```python
from build123d import *

# Parameters (mm, degrees)
CROQUIS1_R                                           = 1.5
CROQUIS1_R_2                                         = 1.75
CROQUIS1_W                                           = 8.011123414
CROQUIS1_H                                           = 3.391601998
CROQUIS1_R_3                                         = 1.642596358
SALIENTE_EXTRUIR1_DEPTH                              = 5
REFRENTADO_PARA_TORNILLO_TAP_N_CON_CABEZ_D           = 3.2
REFRENTADO_PARA_TORNILLO_TAP_N_CON_CABEZ_CSINK_D     = 4.72
REFRENTADO_PARA_TORNILLO_TAP_N_CON_CABEZ_CSINK_ANGLE = 90
REFRENTADO_PARA_TORNILLO_TAP_N_CON_C_2_D             = 3.2
REFRENTADO_PARA_TORNILLO_TAP_N_CON_C_2_CSINK_D       = 6.72
REFRENTADO_PARA_TORNILLO_TAP_N_CON_C_2_CSINK_ANGLE   = 90
CROQUIS7_W                                           = 8
CROQUIS7_H                                           = 13.5
CORTAR_EXTRUIR1_DEPTH                                = 3
CROQUIS8_W                                           = 8
CROQUIS8_H                                           = 2.993534549
CORTAR_EXTRUIR2_DEPTH                                = 10


with BuildPart() as part:
    # Croquis1 → Saliente-Extruir1 (new body)
    with BuildSketch(Plane(origin=(0, 0, 0), x_dir=(1, 0, 0), z_dir=(0, 1, 0))):
        Polygon((-26, 8.5), (-50, 8.5), (-50, -37.5), (50, -37.5), (50, 8.5), (26, 8.5), (26, 37.5), (-26, 37.5), align=None)
        with Locations(Location((-47.484488335, -31.135629499, 0), (0, 0, 270))):
            Circle(CROQUIS1_R, mode=Mode.SUBTRACT)
        with Locations(Location((-47.484488335, -18.135629499, 0), (0, 0, 270))):
            Circle(CROQUIS1_R, mode=Mode.SUBTRACT)
        with Locations(Location((0, -9.329285485, 0), (0, 0, 270))):
            Circle(CROQUIS1_R_2, mode=Mode.SUBTRACT)
        with Locations(Location((47.484488335, -31.135629499, 0), (0, 0, 270))):
            Circle(CROQUIS1_R, mode=Mode.SUBTRACT)
        with Locations(Location((47.484488335, -18.135629499, 0), (0, 0, 270))):
            Circle(CROQUIS1_R, mode=Mode.SUBTRACT)
        with Locations(Location((-47.484488335, -4.135629499, 0), (0, 0, 270))):
            Circle(CROQUIS1_R, mode=Mode.SUBTRACT)
        with Locations(Location((-28.55, -1.504051409, 0), (0, 0, 270))):
            Circle(CROQUIS1_R_2, mode=Mode.SUBTRACT)
        with Locations(Location((0, -1.504051409, 0), (0, 0, 270))):
            Circle(CROQUIS1_R_2, mode=Mode.SUBTRACT)
        with Locations(Location((-21.691369475, 15.250012243, 0), (0, 0, 270))):
            Circle(CROQUIS1_R, mode=Mode.SUBTRACT)
        with Locations(Location((-21.670375076, 33.25, 0), (0, 0, 270))):
            Circle(CROQUIS1_R, mode=Mode.SUBTRACT)
        with Locations(Location((21.691369475, 15.250012243, 0), (0, 0, 270))):
            Circle(CROQUIS1_R, mode=Mode.SUBTRACT)
        with Locations(Location((28.55, -1.504051409, 0), (0, 0, 270))):
            Circle(CROQUIS1_R_2, mode=Mode.SUBTRACT)
        with Locations(Location((47.484488335, -4.135629499, 0), (0, 0, 270))):
            Circle(CROQUIS1_R, mode=Mode.SUBTRACT)
        with Locations((0.009339911, 25.460705384)):
            Rectangle(CROQUIS1_W, CROQUIS1_H, mode=Mode.SUBTRACT)
        with Locations(Location((0.044450606, 34.53510664, 0), (0, 0, 270))):
            Circle(CROQUIS1_R_3, mode=Mode.SUBTRACT)
        with Locations(Location((21.670375076, 33.25, 0), (0, 0, 270))):
            Circle(CROQUIS1_R, mode=Mode.SUBTRACT)
    extrude(amount=SALIENTE_EXTRUIR1_DEPTH)

    # Refrentado para tornillo tap_n con cabez (through all)
    with Locations(Plane(origin=(47.484488335, 0, 4.135629499), x_dir=(0, 0, -1), z_dir=(0, -1, 0))):
        with Locations((0, 0), (-14, 0), (-27, 0), (-27, -94.96897667), (-14, -94.96897667), (0, -94.96897667), (19.385641742, -69.17585781), (19.385641742, -25.79311886), (37.385629499, -25.814113259), (38.670736139, -47.440037729), (37.385629499, -69.154863411)):
            CounterSinkHole(REFRENTADO_PARA_TORNILLO_TAP_N_CON_CABEZ_D / 2, REFRENTADO_PARA_TORNILLO_TAP_N_CON_CABEZ_CSINK_D / 2, counter_sink_angle=REFRENTADO_PARA_TORNILLO_TAP_N_CON_CABEZ_CSINK_ANGLE)

    # Refrentado para tornillo tap_n con c 2 (through all)
    with Locations(Plane(origin=(28.55, 0, 1.504051409), x_dir=(0, 0, -1), z_dir=(0, -1, 0))):
        with Locations((0, 0), (-7.825234076, -28.55), (0, -28.55), (0, -57.1)):
            CounterSinkHole(REFRENTADO_PARA_TORNILLO_TAP_N_CON_C_2_D / 2, REFRENTADO_PARA_TORNILLO_TAP_N_CON_C_2_CSINK_D / 2, counter_sink_angle=REFRENTADO_PARA_TORNILLO_TAP_N_CON_C_2_CSINK_ANGLE)

    # Croquis7 → Cortar-Extruir1 (cut)
    with BuildSketch(Plane.XZ):
        with Locations((-33.626890672, 28.94005161)):
            Rectangle(CROQUIS7_W, CROQUIS7_H)
        with Locations((0, -30.4)):
            Rectangle(CROQUIS7_W, CROQUIS7_H)
        with Locations((33.626890672, 28.94005161)):
            Rectangle(CROQUIS7_W, CROQUIS7_H)
    extrude(amount=-CORTAR_EXTRUIR1_DEPTH, mode=Mode.SUBTRACT)

    # Croquis8 → Cortar-Extruir2 (cut)
    with BuildSketch(Plane.XZ.offset(-3)):
        with Locations((-33.626890672, 34.193284336)):
            Rectangle(CROQUIS8_W, CROQUIS8_H)
        with Locations((33.626890672, 34.193284336)):
            Rectangle(CROQUIS8_W, CROQUIS8_H)
    extrude(amount=-CORTAR_EXTRUIR2_DEPTH, mode=Mode.SUBTRACT)


solid = part.part
```
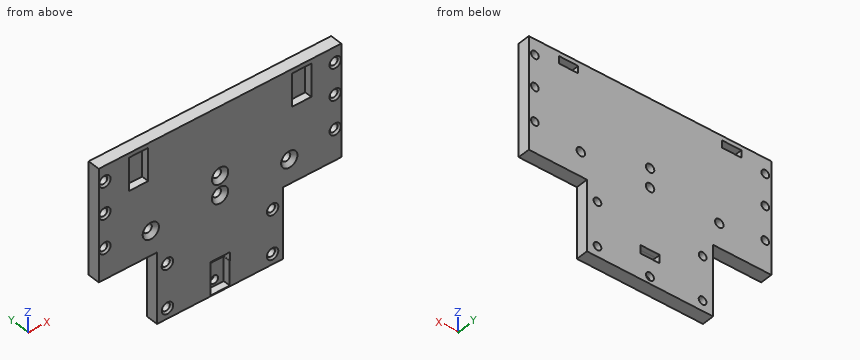
The listing builds one solid part. Answer for the finished solid, in the listing's coordinates (mm). Coordinates: 2 decimals unless noted, no trailing zeros. Write each loop counter-clockwise with the first axis right and the second up, starting at its lowest first coordinate (ties: lowest second). Pieces come first, ordered by that corner, then holes. Notation, with made-up numbers: (22, -33.5) - (34, -33.5) arc R36 ccw to (34, 3.5) - close; hole circle Ø4 at (56, 85). An arc over 180 degrees is marked (long way). Return JSON: item names as keys, results as strings. Group by question number.
1. Given pin 1 (1.7 mm diameter, centred on y = 3.5, z = -25.5, fed in from -X); pin 2 (3 mm diameter, centred on x = 37, y = 2.5, fed in from -Z), each flat-ended and moving along its own axis, determine where each tip first touches the part or whether it passes through.
2. A cutting plane is placed at A-A, the plane x = -28.55. Determine the outline of the cut face in (y, z).
3. A cutting plane is placed at B-B, the plane z = -29.5. Determine the outline of the cut face in (x, y), plus the area to 3 significant figures.
4. A cutting plane is placed at C-C, the plane x = 39. Determine the outline of the cut face in (y, z).
5. Straight lines are drawn through the part: L1, parallel to X at y = 4.15, z = 34; L2, parallel to Z at x = -2, y = 0.9; L3, parallel to X at y = 1.8, z = 19.5. For each, find the intervals that lie inside material, in ascending order.
Ans:
{
 "1": {"pin 1": "x = -26", "pin 2": "z = -8.5"},
 "2": {"outline": "(0, -8.5) - (5, -8.5) - (5, -0.25) - (1.61, -0.25) - (0, -1.86) - close; (0, 4.86) - (1.61, 3.25) - (5, 3.25) - (5, 37.5) - (0, 37.5) - close"},
 "3": {"outline": "(-26, 0) - (-4, 0) - (-4, 3) - (4, 3) - (4, 0) - (26, 0) - (26, 5) - (-26, 5) - close", "area": "236 mm²"},
 "4": {"outline": "(0, -8.5) - (5, -8.5) - (5, 37.5) - (0, 37.5) - close"},
 "5": {"L1": "-50 to -37.63, -29.63 to 29.63, 37.63 to 50", "L2": "-37.5 to -37.15, -23.65 to 0.07, 2.94 to 7.9, 10.76 to 37.5", "L3": "-50 to -48.32, -46.65 to 46.65, 48.32 to 50"}
}
